from build123d import *

# Parameters (mm, degrees)
F0_R     = 7.5
F1_DEPTH = 2
F2_R     = 2.5
F3_DEPTH = 56.4


with BuildPart() as f1:
    # F0 (on Top) → F1 (new body)
    with BuildSketch(Plane.XY):
        Circle(F0_R)
    extrude(amount=F1_DEPTH)

    # F2 (on Top) → F3 (join)
    with BuildSketch(Plane.XY):
        Circle(F2_R)
    extrude(amount=F3_DEPTH)

    # F4 (on Front) → F5 (revolve)
    with BuildSketch(Plane.XZ):
        Polygon((-2.470695, 56.377843), (0, 56.377843), (2.45018, 56.377843), (0, 60.79717), align=None)
    revolve(axis=Axis((1.22509, 0, 56.377843), (1, 0, 0)))


solid = f1.part
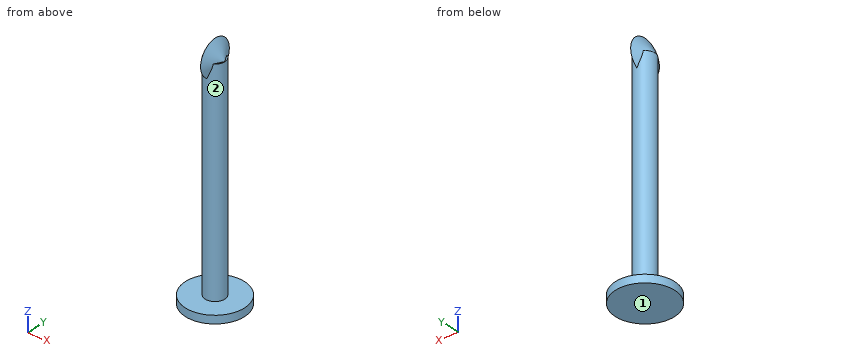
The model under review builds one solid part; all positions refer to its coordinate system, in mm. Face numbers are marked on the shaded views. A direction names the side the tool comes from. Coordinates: 2 decimals unless noted, no trailing zeros. Order: outer loops, then holes, each group sorted by start corner. A loop starts at its lowest first (then second) coordinate and runs counter-clockwise, first axis right, second up. Notation, with made-up numbers: (46.25, 3.25) -> (85.25, 3.25) arc R27 cw to (85.25, 39.25) -> close; hole circle Ø5 at (-25, -34.5). An arc over 180 degrees is marked (long way). Answer in a Markdown table with one row per item.
(1) Insertion check: pin 1 (1.4 mm diameter, centred on x = -2, y = 0, fed in from +Z); pin 2 (2 mm diameter, centred on x = -5.5, y = -2, fed in from +Z); pin 3 (0.6 mm diameter, centred on x = 1.5, y = 0, fed in from +Z). Each pin has a flat end and moves straight along its axis. Give the tip position at first contact, or say it passes through.
Answers:
| item | result |
|---|---|
| pin 1 | z = 58.47 |
| pin 2 | z = 2 |
| pin 3 | z = 58.63 |
(2) Wall thickness on line 1 along Y through (x, z) = (0.25, 43.5); line 2 along X through (y, z) = (0.5, 40.5); line 3 along Z through (x, y) = (3, -6.5): over which ranges is each line inside the solid? List them lowest first.
Answers:
| item | result |
|---|---|
| line 1 | -2.49 to 2.49 |
| line 2 | -2.45 to 2.45 |
| line 3 | 0 to 2 |
(3) Machinability: for the marked faces 1 and 2, which of the approach directions +Z, -Z, +X, -X, +Y, -Y give a long, thin tool a straight path to every point of the face, cutting with its end or side? Answer none if there is none.
Answers:
| item | result |
|---|---|
| face 1 | -Z, +X, -X, +Y, -Y |
| face 2 | none |
(4) Consider section A-A (y = 0). Write out the cut boundary in (x, z).
Answers:
| item | result |
|---|---|
| outline | (-7.5, 0) -> (7.5, 0) -> (7.5, 2) -> (2.5, 2) -> (2.5, 56.4) -> (2.44, 56.4) -> (0, 60.8) -> (-2.46, 56.4) -> (-2.5, 56.4) -> (-2.5, 2) -> (-7.5, 2) -> close |
(5) Consider section D-D (y = -5). Write out the cut boundary in (x, z), plus the area to 3 significant figures.
Answers:
| item | result |
|---|---|
| outline | (-5.59, 0) -> (5.59, 0) -> (5.59, 2) -> (-5.59, 2) -> close |
| area | 22.4 mm² |
(6) Consider section C-C (x = 4.25). Write out the cut boundary in (y, z).
Answers:
| item | result |
|---|---|
| outline | (-6.18, 0) -> (6.18, 0) -> (6.18, 2) -> (-6.18, 2) -> close |
(7) Consider section B-B (z = 23). Write out the cut boundary in (x, y), plus the area to 3 significant figures.
Answers:
| item | result |
|---|---|
| outline | circle Ø5 at (0, 0) |
| area | 19.6 mm² |
